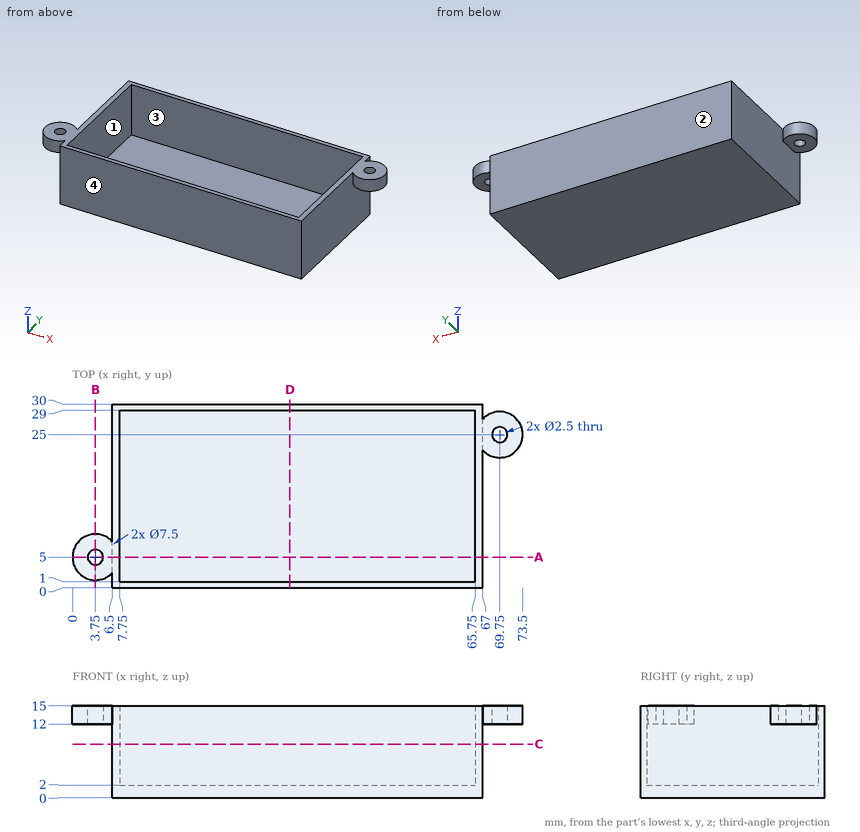
Here's the drawing with two shaded views (mm, measured from the low corner). I have some questions. A direction names the side the tool comes from. Round coordinates to 2 decimals unless told otherwise and drop trailing zeros. Loops run counter-clockwise (first coordinate to the right, second up) from the corner with the lowest first, then second, coordinate; pieces in that order, holes last. Notation, with made-up numbers: (47.5, 0.25) -> (83.5, 0.25) arc R18 ccw to (83.5, 14.25) -> close; hole circle Ø3 at (27.5, -26.5). An arc over 180 degrees is marked (long way). Answer as CSV lines item,"result". Start each with the question number.
1. For the marked faces 1 and 2, which set-ups out of +Z, -Z, +X, -X, +Y, -Y let a thin tool reach every point of the face, with its end or its side?
2. Imagine slicing it at B-B on x = 3.75. Write out the boundary of the cut face in (y, z).
3. I need wall thicknesses on probe 1 along Y at (x, z) = (69.75, 14.3); probe 2 along Y at (x, z) = (51, 13.25); probe 3 along X at (y, z) = (9.75, 8.25). Which ranges of each line are inside material? Lowest first, please. Write a range as from..to.
4. Imagine slicing it at A-A on y = 5. Write out the boundary of the cut face in (x, z).
5. If we mould it in two halves opening along X, with no side actions, what happens to the marked faces 3 and 4? For each: pulls with the +X half, pulls with the -X half, needs draft (parallel to the pull), parting line crosses it, or undercut.
6. Imagine slicing it at D-D on x = 35.5. Write out the boundary of the cut face in (y, z), plus the area to 3 significant figures.
7. Imagine slicing it at C-C on z = 8.75. Write out the boundary of the cut face in (x, y).
8. I'm going to push flat-ended pins straight in: P1, Ø3, axis at x = 69.75, y = 25, coming from the -Z side; P2, Ø7.5, axis at y = 15.5, z = 5, coming from the +X side; P3, Ø6.5, axis at y = 8.5, z = 8.5, coming from the -X side. Where does each tip first touch, or does it pass through?
Solution:
1,face 1,"+Z"
1,face 2,"+Z, -Z, +X, -X, +Y"
2,outline,"(1.25, 12) -> (3.75, 12) -> (3.75, 15) -> (1.25, 15) -> close; (6.25, 12) -> (8.75, 12) -> (8.75, 15) -> (6.25, 15) -> close"
3,probe 1,"21.25..23.75, 26.25..28.75"
3,probe 2,"0..1, 29..30"
3,probe 3,"6.5..7.75, 65.75..67"
4,outline,"(0, 12) -> (2.5, 12) -> (2.5, 15) -> (0, 15) -> close; (5, 12) -> (6.5, 12) -> (6.5, 0) -> (67, 0) -> (67, 15) -> (65.75, 15) -> (65.75, 2) -> (7.75, 2) -> (7.75, 15) -> (5, 15) -> close"
5,face 3,"undercut"
5,face 4,"needs draft"
6,outline,"(0, 0) -> (30, 0) -> (30, 15) -> (29, 15) -> (29, 2) -> (1, 2) -> (1, 15) -> (0, 15) -> close"
6,area,"86.0 mm²"
7,outline,"(6.5, 0) -> (67, 0) -> (67, 30) -> (6.5, 30) -> close; hole (7.75, 1) -> (65.75, 1) -> (65.75, 29) -> (7.75, 29) -> close"
8,P1,"z = 12"
8,P2,"x = 67"
8,P3,"x = 6.5"
